For this review, take the finished solid that the model builds, in its own axes (mm). A direction names the side the tool comes from. Round coordinates to 2 decimals unless told otherwise and drop trailing zeros. Order: outer loops, then holes, each group sorted by start corner. A loop starts at its lowest first (then second) coordinate and runs counter-clockwise, first axis right, second up.
```python
from build123d import *

# Parameters (mm, degrees)
F1_DEPTH    = 38.1
F3_DEPTH    = 76.2
F5_DEPTH    = 76.201
F6_T1_DEPTH = 76.2
F6_T3_DEPTH = 101.6
F7_R        = 10.16
F8_SIZE     = 5.08
F9_R        = 8.89


# Not quite as in the source:
# - a fillet or chamfer that OpenCascade refuses, or shapes differently, is made with other operations: its cross-section is extruded or revolved along the edge and cut away or added


with BuildPart() as f1:
    # F0 (on Right) → F1 (new body, symmetric)
    with BuildSketch(Plane.YZ):
        Polygon((-12.7, 31.75), (-12.7, 0), (12.7, 0), (56.6940905122, 76.2), (76.2, 76.2), (76.2, 0), (85.725, 0), (85.725, 85.725), (51.1948291982, 85.725), (12.7, 19.05), (7.200738686, 9.525), (-3.175, 9.525), (-3.175, 19.05), (-3.175, 31.75), align=None)
        Polygon((12.7, 19.05), (-3.175, 19.05), (-3.175, 9.525), (7.200738686, 9.525), align=None)
    extrude(amount=F1_DEPTH, both=True)

    # F2 (on face) → F3 (join, through all)
    with BuildSketch(Plane.YZ.offset(38.1)):
        Polygon((56.6940905122, 76.2), (12.7, 0), (76.2, 0), (76.2, 76.2), align=None)
    extrude(amount=-F3_DEPTH)

    # F4 (on face) → F5 (cut, through all)
    with BuildSketch(Plane.YZ.offset(38.1)):
        Polygon((58.5271776169, 73.025), (23.6985226281, 12.7), (73.025, 12.7), (73.025, 73.025), align=None)
    extrude(amount=-F5_DEPTH, mode=Mode.SUBTRACT)

    # F6: fillet of radius 5.08 on 3 edges, made by hand

    # F6_s2 → F6_t1 (join)
    with BuildSketch(Plane.YZ.offset(-38.1)):
        with BuildLine():
            ThreePointArc((-3.175, 24.13), (-1.6871024484, 20.5378975516), (1.905, 19.05))
            Line((1.905, 19.05), (-3.175, 19.05))
            Line((-3.175, 19.05), (-3.175, 24.13))
        make_face()
    extrude(amount=F6_T1_DEPTH)

    # F6_s4 → F6_t3 (cut)
    with BuildSketch(Plane.YZ.offset(-50.8)):
        with BuildLine():
            ThreePointArc((-3.175, 26.67), (-4.6628975516, 30.2621024484), (-8.255, 31.75))
            Line((-8.255, 31.75), (-3.175, 31.75))
            Line((-3.175, 31.75), (-3.175, 26.67))
        make_face()
        with BuildLine():
            ThreePointArc((-7.62, 31.75), (-11.2121024484, 30.2621024484), (-12.7, 26.67))
            Line((-12.7, 26.67), (-12.7, 31.75))
            Line((-12.7, 31.75), (-7.62, 31.75))
        make_face()
    extrude(amount=F6_T3_DEPTH, mode=Mode.SUBTRACT)

    # F7
    f7_edges = [f1.edges().sort_by_distance(p)[0] for p in [
        (0, 12.7, 19.05),
        (0, 51.194829, 85.725),
        (0, 85.725, 85.725),
        (0, 23.698523, 12.7),
        (0, 73.025, 12.7),
    ]]
    fillet(f7_edges, radius=F7_R)

    # F8
    f8_edges = [f1.edges().sort_by_distance(p)[0] for p in [
        (0, 85.725, 0),
        (0, -12.7, 0),
    ]]
    chamfer(f8_edges, length=F8_SIZE)

    # F9
    f9_edges = [f1.edges().sort_by_distance(p)[0] for p in [
        (0, 73.025, 73.025),
        (0, 58.527178, 73.025),
    ]]
    fillet(f9_edges, radius=F9_R)


solid = f1.part
```
Q1. Take a section at D-D, the plane y = 20.5. State the section outline as (x, z) points, plus the area to 3 significant figures.
Q2. Mouldability with a two-part tool opening along Y and no side actions: class faces 4 (the face through (0.53, 51.92, 84.33)), 5 (the face through (1, 73.025, 43)), 6 (the face through (1, 66, 85.725)), 7 (the face through (1, 85.725, 40)) as +Y half, -Y half, draft (parallel to the pull), parting line (faces both ways), or undercut.
Q3. Clearance check with flat-ended pins moving along their axes: pin 1 (2 mm diameter, centred on x = 13, y = 35, fed in from +Z); pin 2 (5 mm diameter, centred on y = 37, z = 62.5, fed in from +X); pin 3 (8 mm diameter, centred on x = -7.5, y = 12, fed in from +Z); pin 4 (5.5 mm diameter, centred on x = -14.5, y = 4, fed in from +Z). State where each tip first meets the part, or that it passes through.
Q4. Take a section at B-B, the plane y = 70. State the section outline as (x, z) points (3 decimals), plus the area to 3 significant figures.
Q5. Wall thickness on line 1 (Z direction, x = -20, y = 63.5) (3 decimals); line 2 (Y direction, x = -4, z = 60.5) (3 decimals); line 3 (Z direction, x = 16, y = 60) (3 decimals): over which ranges is each line inside the solid? List them lowest first.
Q6. Take a section at C-C, the plane z = 54.5. State the section outline as (x, y) points (3 decimals), plus the area to 3 significant figures.
Q7. Tool access review of faces 1 (the face through (0.533, 11.849, 20.374)), 2 (the face through (0.5, 82.8, 82.7)), 3 (the face through (0.53, 44.39, 48.54)): name each direction out of +Z, -Z, +X, -X, +Y, -Y from which nothing blocks a thin tool from reaching the whole face with its end or side.
Working result:
1. outline: (-38.1, 0) - (38.1, 0) - (38.1, 32.56) - (-38.1, 32.56) - close
1. area: 2,480 mm2
2. face 4: -Y half
2. face 5: undercut
2. face 6: draft
2. face 7: +Y half
3. pin 1: stops at z = 59.41
3. pin 2: stops at x = 38.1
3. pin 3: stops at z = 24.77
3. pin 4: stops at z = 19.09
4. outline: (-38.1, 0) - (38.1, 0) - (38.1, 15.627) - (-38.1, 15.627) - close; (-38.1, 70.816) - (38.1, 70.816) - (38.1, 85.725) - (-38.1, 85.725) - close
4. area: 2,330 mm2
5. line 1: z = 0 to 12.72, 73.024 to 85.725
5. line 2: y = 36.631 to 51.296, 73.025 to 85.725
5. line 3: z = 0 to 12.7, 72.237 to 85.725
6. outline: (-38.1, 33.167) - (38.1, 33.167) - (38.1, 47.832) - (-38.1, 47.832) - close; (-38.1, 73.025) - (38.1, 73.025) - (38.1, 85.725) - (-38.1, 85.725) - close
6. area: 2,090 mm2
7. face 1: +Z, +X, -X
7. face 2: +Z, +X, -X, +Y
7. face 3: +X, -X
